Geometry: see drawing. Coordinates: mm, zero at the bounding-box minimum. A direction names the side the tool comes from. Coordinates: 2 decimals unless noted, no trailing zeros. Loops run counter-clockwise (first coordinate to the right, second up) from the corner with the lowest first, then second, coordinate; pieces in that order, holes last. Notation, with made-up numbers: M 68.5,-32 L 114.5,-32 A23 cw 114.5,-6 Z; hole C -6,89 d10. An arc over 180 degrees is marked long. Write each question's results on one line, items separated by ' | '. Start each with the question number.
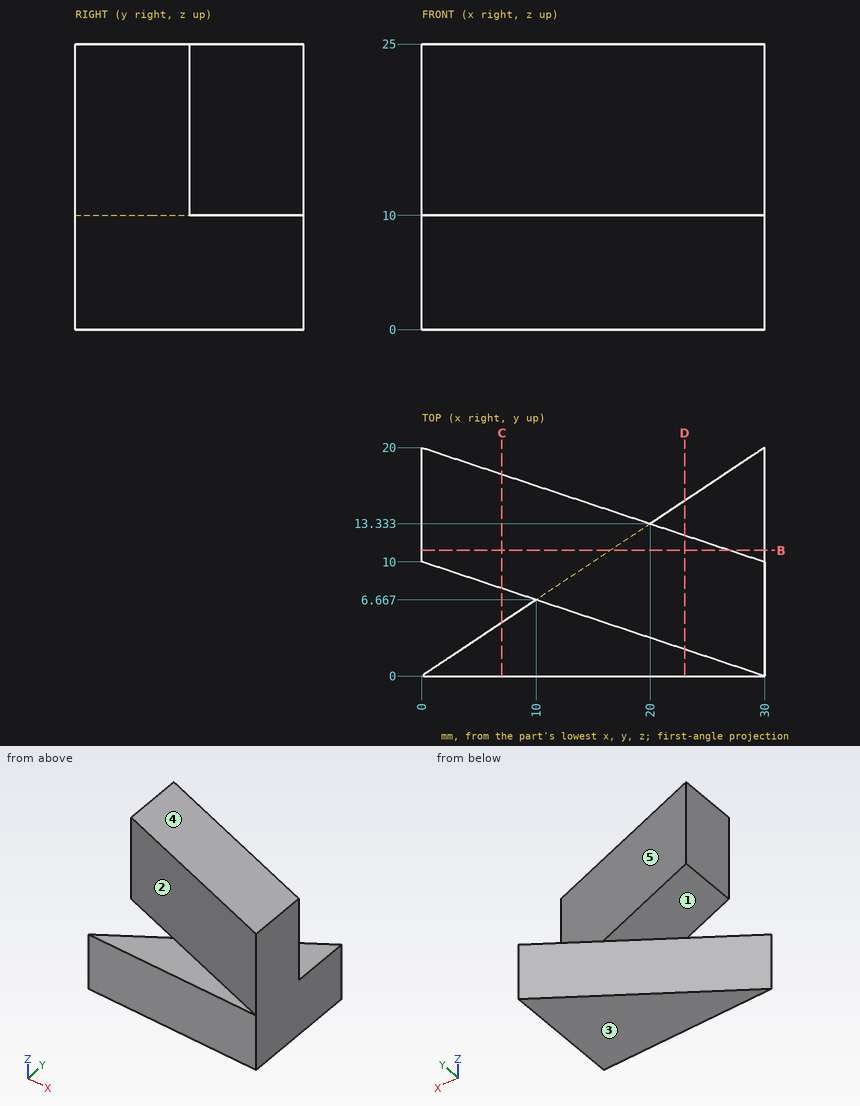
Item 1: Cut plane D-D (x = 23). Output: boundary loops of the cut face in (y, z), then the cut area to 3 significant figures.
Item 2: First-contact query: pin 1 Ø10 at (x, z) = (20, 13) entering from +Y; pin 2 Ø10.5 at (x, y) = (12, 16) entering from -Z; pin 3 Ø1 at (y, z) = (8, 4) entering from -X. Flat tips, straight axial feed; report the tip coordinate or a pass-through.
Item 3: Cut plane C-C (x = 7). Output: boundary loops of the cut face in (y, z), then the cut area to 3 significant figures.
Item 4: Line query: probe 1 along Z at (x, y) = (5, 17.5); probe 2 along Z at (x, y) = (12, 1.5); probe 3 along Y at (x, z) = (19, 13). Output: solid intervals per line, ascending.
Item 5: Cut plane B-B (y = 11). Output: boundary loops of the cut face in (x, z).
Item 6: Access query for the marked faces 1, 2, 3, 4 and 5. Directions: +Z, -Z, +X, -X, +Y, -Y. A direction counts if a zero-diameter tool reaches every point of the face in a straight line with its end or side. Return the directions, or none.
Response values:
1) outline: M 0,0 L 15.33,0 L 15.33,10 L 12.33,10 L 12.33,25 L 2.33,25 L 2.33,10 L 0,10 Z | area: 303 mm2
2) pin 1: stops at y = 16 | pin 2: stops at z = 10 | pin 3: stops at x = 11.25
3) outline: M 0,0 L 4.67,0 L 4.67,10 L 0,10 Z; M 7.67,10 L 17.67,10 L 17.67,25 L 7.67,25 Z | area: 197 mm2
4) probe 1: z = 10 to 25 | probe 2: z = 0 to 10 | probe 3: y = 3.67 to 13.67
5) outline: M 0,10 L 16.5,10 L 16.5,0 L 30,0 L 30,10 L 27,10 L 27,25 L 0,25 Z
6) face 1: -Z, -X, +Y | face 2: +Z, -X, -Y | face 3: -Z, +X, -X, +Y, -Y | face 4: +Z, +X, -X, +Y, -Y | face 5: +Z, +X, +Y
